from build123d import *

# Parameters (mm, degrees)
SKETCH1_W           = 6
SKETCH1_H           = 6
BOSS_EXTRUDE1_DEPTH = 33
SKETCH2_R           = 2
CUT_EXTRUDE1_DEPTH  = 33
SKETCH3_W           = 6
SKETCH3_H           = 15
BOSS_EXTRUDE2_DEPTH = 1.5


with BuildPart() as part:
    # Sketch1 → Boss-Extrude1 (new body)
    with BuildSketch(Plane(origin=(0, 0, 0), x_dir=(1, 0, 0), z_dir=(0, 1, 0))):
        Rectangle(SKETCH1_W, SKETCH1_H)
    extrude(amount=BOSS_EXTRUDE1_DEPTH)

    # Sketch2 → Cut-Extrude1 (cut)
    with BuildSketch(Plane.XY.offset(3)):
        with Locations((0, 28.5)):
            Circle(SKETCH2_R)
        with Locations((0, 4.5)):
            Circle(SKETCH2_R)
    extrude(amount=-CUT_EXTRUDE1_DEPTH, mode=Mode.SUBTRACT)

    # Sketch3 → Boss-Extrude2 (add)
    with BuildSketch(Plane(origin=(3, 0, 0), x_dir=(0, 0, -1), z_dir=(1, 0, 0))):
        with Locations((0, 7.5)):
            Rectangle(SKETCH3_W, SKETCH3_H)
    extrude(amount=BOSS_EXTRUDE2_DEPTH)


solid = part.part
Part model, mm, in its own coordinate system. A direction names the side the tool comes from. Give positions to 0.01 mm unless a question says otherwise; leave off trailing zeros. Order: outer loops, then holes, each group sorted by start corner. A loop starts at its lowest first (then second) coordinate and runs counter-clockwise, first axis right, second up. Notation, with made-up numbers: (-12.75, 0.25) - (34.25, 0.25) arc R21 cw to (34.25, 24.25) - close; hole circle Ø4 at (-20, 38). An arc over 180 degrees is marked (long way). Use a Markdown table: item, result.
1) 3-axis set-ups, long thin cutter, end or side, ignore diameter. For faces 5 (the flat face through (-3, 16, 0)), 6 (the flat face through (4, 15, 0)): which of +Z, -Z, +X, -X, +Y, -Y reach the whole face in a straight line?
Checked values:
| item | result |
|---|---|
| face 5 | +Z, -Z, -X, +Y, -Y |
| face 6 | +Z, -Z, +X, +Y |
2) Probe L1, parallel to Y at x = 0, z = 0.7; L2, parallel to Y at x = 0.5, z = 1.45; L3, parallel to X at y = 31.5, z = 2.7. List the from-to ranges inside material, lowest first. Write a range as from..to.
Checked values:
| item | result |
|---|---|
| L1 | 0..2.5, 6.5..26.5, 30.5..33 |
| L2 | 0..2.56, 6.44..26.56, 30.44..33 |
| L3 | -3..3 |
3) Flat gauge pins, fed straight in: P1, Ø1.8, axis at y = 23, z = 1, coming from the +X side; P2, Ø1.6, axis at x = 4, z = 1, coming from the +Y side; P3, Ø3, axis at x = 0, y = 4.5, coming from the +Z side. Where does each tip first touch, or does it go through?
Checked values:
| item | result |
|---|---|
| P1 | x = 3 |
| P2 | y = 15 |
| P3 | through |
4) Two-plate mould, pull along Y, no slides. Class faces 1 (the flat face through (3, 24, 0)), 2 (the cylindrical face through (-0.434, 2.548, 0.042)), 3 (the flat face through (1, 0, 0)), 4 (the flat face through (0, 33, 0)): +Y half, -Y half, draft (parallel to the pull), parting line (faces both ways), or undercut.
Checked values:
| item | result |
|---|---|
| face 1 | draft |
| face 2 | undercut |
| face 3 | -Y half |
| face 4 | +Y half |
5) Saw through at A-A on y = 28.5. List the corners of the cut face in (x, z).
Checked values:
| item | result |
|---|---|
| outline | (-3, -3) - (-2, -3) - (-2, 3) - (-3, 3) - close; (2, -3) - (3, -3) - (3, 3) - (2, 3) - close |
6) Saw through at B-B on x = 0. List the corners of the cut face in (y, z).
Checked values:
| item | result |
|---|---|
| outline | (0, -3) - (2.5, -3) - (2.5, 3) - (0, 3) - close; (6.5, -3) - (26.5, -3) - (26.5, 3) - (6.5, 3) - close; (30.5, -3) - (33, -3) - (33, 3) - (30.5, 3) - close |
7) Saw through at C-C on z = -0.85. List the corners of the cut face in (x, y), plus the area to 3 significant figures.
Checked values:
| item | result |
|---|---|
| outline | (-3, 0) - (4.5, 0) - (4.5, 15) - (3, 15) - (3, 33) - (-3, 33) - close; hole circle Ø4 at (0, 4.5); hole circle Ø4 at (0, 28.5) |
| area | 195 mm² |
8) Saw through at D-D on y = 4.5. List the corners of the cut face in (x, z), plus the area to 3 significant figures.
Checked values:
| item | result |
|---|---|
| outline | (-3, -3) - (-2, -3) - (-2, 3) - (-3, 3) - close; (2, -3) - (4.5, -3) - (4.5, 3) - (2, 3) - close |
| area | 21.0 mm² |
